Autodesk Inventor part; units mm, degrees
ref_plane "YZ Plane" through (0, 0, 0) normal (1, 0, 0) x (0, 1, 0)
ref_plane "XZ Plane" through (0, 0, 0) normal (0, 1, 0) x (-1, 0, 0)
ref_plane "XY Plane" through (0, 0, 0) normal (0, 0, 1) x (1, 0, 0)
sketch "Sketch1" plane through (0, 0, 0) normal (0, 0, 1) x (1, 0, 0)
  circle A0 centre (9.525, -12.7) radius 3.3782
  line L0 (19.05, 0) -> (0, 0)
  line L1 (0, 0) -> (0, -25.4)
  line L2 (19.05, -25.4) -> (0, -25.4)
  line L3 (19.05, 0) -> (19.05, -25.4)
extrude "Plate1" add sketch "Sketch1" along normal blind 3.175
sketch "Sketch2" plane through (19.05, -22.225, 0) normal (0, -1, 0) x (1, 0, 0)
  line L0 (-19.05, 0) -> (0, 0)
  line L1 (0, 0) -> (0, 25.4)
  line L2 (0, 25.4) -> (-19.05, 25.4)
  line L3 (-19.05, 25.4) -> (-19.05, 0)
edge flange "Flange1" height 25.4 angle 90 thickness 3.175 bend radius 1.27 thickness toward (0, -1, 0) relief straight relief width 3.175 relief depth 1.5875 edges at (9.525, -25.4, 3.175) wall of the first edge with corners at (0, -22.225, 0) (19.05, -22.225, 0) (19.05, -22.225, 25.4) (0, -22.225, 25.4)
bend "Bend1"
corner "Corner1"
sketch "Sketch3" plane through (0, -25.4, 25.4) normal (0, 0, 1) x (1, 0, 0)
  line L0 (0, 0) -> (19.05, 0)
  line L1 (19.05, 3.175) -> (19.05, 0)
  line L2 (0, 3.175) -> (19.05, 3.175)
  line L3 (0, 3.175) -> (0, 0)
  point P0 (0, 25.4)
extrude "Extrusion1" add sketch "Sketch3" along normal blind 25.4
equation "\"d1\" = BendReliefWidth"
equation "\"d2\" = BendReliefDepth"
equation "\"d3\" = MinimumRemnant"
equation "\"d4\" = BendRadius"
equation "\"d8\" = CornerReliefSize"
equation "\"d9\" = GapSize"
equation "\"d10\" = JacobiRadiusSize"
equation "\"BendRadius\" = Thickness"
equation "\"BendReliefWidth\" = Thickness"
equation "\"BendReliefDepth\" = 0.5 * Thickness"
equation "\"CornerReliefSize\" = 4 * Thickness"
equation "\"MinimumRemnant\" = 2 * Thickness"
equation "\"TransitionRadius\" = BendRadius"
equation "\"JacobiRadiusSize\" = Thickness"
equation "\"GapSize\" = Thickness"
equation "\"d0\" = BendRadius"
Read the model definition and answer for the solid it produces. Units are mm, in the model's axes. A direction names the side the tool comes from. Give positions to 0.01 mm unless a question says otherwise; leave off trailing zeros. Loops run counter-clockwise (first coordinate to the right, second up) from the corner with the lowest first, then second, coordinate; pieces in that order, holes last. Notation, with made-up numbers: M 75,18.5 L 106,18.5 A22 cw 106,30.5 Z; hole C 35,79 d2. An arc over 180 degrees is marked long. Write each question's results on one line, items separated by ' | '.
1. Section B-B on x = 14 is taken. Give the vertices of the cut face in (y, z) (3 decimals).
Values:
outline: M -25.4,4.445 A4.445 ccw -20.955,0 L 0,0 L 0,3.175 L -20.955,3.175 A1.27 cw -22.225,4.445 L -22.225,50.8 L -25.4,50.8 Z
2. Given pin 1 (8 mm diameter, centred on x = 8, z = 10, fed in from +Y) (3 decimals); pin 2 (5.5 mm diameter, centred on x = 12.5, y = -15, fed in from +Z) (3 decimals), each flat-ended and moving along its own axis, determine where each tip first touches the part or whether it passes through.
Values:
pin 1: stops at y = -22.225 | pin 2: stops at z = 3.175
3. A tool of negligible diameter and unlimited length cuts with its end or side. For faces 5 (the face through (19.05, -23, 18)), 6 (the face through (9, -8, 3.175)), from which of +Z, -Z, +X, -X, +Y, -Y can it reach the whole face along a straight path? Write none if from no direction.
Values:
face 5: +Z, -Z, +X, +Y, -Y | face 6: +Z, +X, -X, +Y
4. Section D-D on z = 43.5 is taken. Give the vertices of the cut face in (x, y) (3 decimals), plus the area to 3 significant figures.
Values:
outline: M 0,-25.4 L 19.05,-25.4 L 19.05,-22.225 L 0,-22.225 Z | area: 60.5 mm^2
5. Section C-C on x = 9.25 is taken. Give the vertices of the cut face in (y, z) (3 decimals), plus the area to 3 significant figures.
Values:
outline: M -25.4,4.445 A4.445 ccw -20.955,0 L -16.067,0 L -16.067,3.175 L -20.955,3.175 A1.27 cw -22.225,4.445 L -22.225,50.8 L -25.4,50.8 Z; M -9.333,0 L 0,0 L 0,3.175 L -9.333,3.175 Z | area: 207 mm^2
6. Section A-A on y = -12.7 is taken. Give the vertices of the cut face in (x, z) (3 decimals).
Values:
outline: M 0,0 L 6.147,0 L 6.147,3.175 L 0,3.175 Z; M 12.903,0 L 19.05,0 L 19.05,3.175 L 12.903,3.175 Z
7. Straight lines are drawn through the part: line 1 (Z direction, x = 3, y = -19.75) (3 decimals); line 2 (Y direction, x = 8.75, z = 4.5) (3 decimals); line 3 (Y direction, x = 10.5, z = 4). For each, find the intervals that lie inside material, in ascending order. Write a range as [from, to].
Values:
line 1: z = [0, 3.175] | line 2: y = [-25.4, -22.225] | line 3: y = [-25.38, -22.14]
8. The mould has two halves that part along Y. Classify faces 1 (the face through (9.658, -24.132, 1.337)), 2 (the face through (6.844, -10.644, 1.565)), 3 (the face through (10, 0, 2)), 4 (the face through (0, -23, 18)): pulls with the +Y half, pulls with the -Y half, needs draft (parallel to the pull), parting line crosses it, or undercut.
Values:
face 1: pulls with the -Y half | face 2: undercut | face 3: pulls with the +Y half | face 4: needs draft
